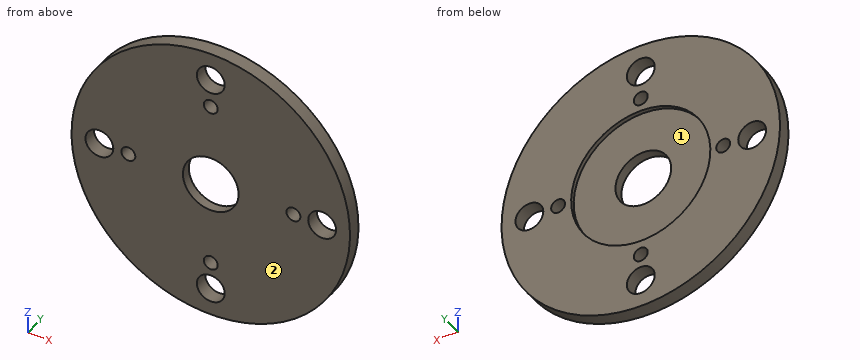
```python
from build123d import *

# Parameters (mm, degrees)
SKETCH1_R           = 10
SKETCH1_R_2         = 2
SKETCH1_R_3         = 1
SKETCH1_R_4         = 0.5
BOSS_EXTRUDE1_DEPTH = 1
SKETCH2_R           = 5
CUT_EXTRUDE1_DEPTH  = 0.3


with BuildPart() as part:
    # Sketch1 → Boss-Extrude1 (new body)
    with BuildSketch(Plane(origin=(0, 0, 0), x_dir=(1, 0, 0), z_dir=(0, 1, 0))):
        with Locations(Location((0, 0, 0), (0, 0, 270))):  # turned: the seam where the file's is
            Circle(SKETCH1_R)
        with Locations(Location((0, 0, 0), (0, 0, 270))):  # turned: the seam where the file's is
            Circle(SKETCH1_R_2, mode=Mode.SUBTRACT)
        with Locations(Location((-8, 0, 0), (0, 0, 270))):  # turned: the seam where the file's is
            Circle(SKETCH1_R_3, mode=Mode.SUBTRACT)
        with Locations(Location((-5.919172613, 0, 0), (0, 0, 270))):  # turned: the seam where the file's is
            Circle(SKETCH1_R_4, mode=Mode.SUBTRACT)
        with Locations(Location((0, -5.941415712, 0), (0, 0, 90))):  # turned: the seam where the file's is
            Circle(SKETCH1_R_4, mode=Mode.SUBTRACT)
        with Locations(Location((0, -8, 0), (0, 0, 90))):  # turned: the seam where the file's is
            Circle(SKETCH1_R_3, mode=Mode.SUBTRACT)
        with Locations(Location((5.936823246, 0, 0), (0, 0, 90))):  # turned: the seam where the file's is
            Circle(SKETCH1_R_4, mode=Mode.SUBTRACT)
        with Locations(Location((8, 0, 0), (0, 0, 90))):  # turned: the seam where the file's is
            Circle(SKETCH1_R_3, mode=Mode.SUBTRACT)
        with Locations(Location((0, 6.0333524, 0), (0, 0, 270))):  # turned: the seam where the file's is
            Circle(SKETCH1_R_4, mode=Mode.SUBTRACT)
        with Locations(Location((0, 8, 0), (0, 0, 270))):  # turned: the seam where the file's is
            Circle(SKETCH1_R_3, mode=Mode.SUBTRACT)
    extrude(amount=BOSS_EXTRUDE1_DEPTH)

    # Sketch2 → Cut-Extrude1 (cut)
    with BuildSketch(Plane(origin=(0, 1, 0), x_dir=(1, 0, 0), z_dir=(0, 1, 0))):
        with Locations(Location((0, 0, 0), (0, 0, 270))):  # turned: the seam where the file's is
            Circle(SKETCH2_R)
    extrude(amount=-CUT_EXTRUDE1_DEPTH, mode=Mode.SUBTRACT)


solid = part.part
```
Here's how the part is built. I have some questions about the finished solid (model axes, mm). Face numbers are marked on the shaded views. Coordinates: 2 decimals unless noted, no trailing zeros. Loops run counter-clockwise (first coordinate to the right, second up) from the corner with the lowest first, then second, coordinate; pieces in that order, holes last. Notation, with made-up numbers: M -30,58.5 L 17,58.5 A26 ccw 17,86.5 Z; hole C 63.25,7.5 d9. An arc over 180 degrees is marked long. One line per item, written item: value.
1. Imagine slicing it at A-A (x = -8). List the corners of the cut face in (y, z) for me, and give its area (3 significant figures).
Geometry says:
outline: M 0,-6 L 1,-6 L 1,-1 L 0,-1 Z; M 0,1 L 1,1 L 1,6 L 0,6 Z
area: 10.0 mm2
2. Will this pin go through, and if not, where does the flat tip stop? pin 1 Ø2.5 at (x, z) = (8, 0) entering from -Y.
Geometry says:
pin 1: stops at y = 0
3. Imagine slicing it at D-D (x = 0). List the corners of the cut face in (y, z) for me, and give its area (3 significant figures).
Geometry says:
outline: M 0,-10 L 1,-10 L 1,-9 L 0,-9 Z; M 0,-7 L 1,-7 L 1,-6.53 L 0,-6.53 Z; M 0,-5.53 L 1,-5.53 L 1,-5 L 0.7,-5 L 0.7,-2 L 0,-2 Z; M 0,2 L 0.7,2 L 0.7,5 L 1,5 L 1,5.44 L 0,5.44 Z; M 0,6.44 L 1,6.44 L 1,7 L 0,7 Z; M 0,9 L 1,9 L 1,10 L 0,10 Z
area: 8.20 mm2
4. Thinking about a two-plate mould opening in Z: for the marked faces 1 and 2, which applies, +Z half, -Z half, draft (parallel to the pull), parting line (faces both ways), or undercut?
Geometry says:
face 1: undercut
face 2: draft
5. Imagine slicing it at C-C (z = 8). List the corners of the cut face in (x, y) for me, and give its area (3 significant figures).
Geometry says:
outline: M -6,0 L -1,0 L -1,1 L -6,1 Z; M 1,0 L 6,0 L 6,1 L 1,1 Z
area: 10.0 mm2
6. Please list where these lines run through material, in increasing order: probe 1 along X at (y, z) = (0.3, 0); probe 2 along X at (y, z) = (0.8, 0); probe 3 along X at (y, z) = (0.95, -6).
Geometry says:
probe 1: x = -10 to -9, -7 to -6.42, -5.42 to -2, 2 to 5.44, 6.44 to 7, 9 to 10
probe 2: x = -10 to -9, -7 to -6.42, -5.42 to -5, 5 to 5.44, 6.44 to 7, 9 to 10
probe 3: x = -8 to -0.5, 0.5 to 8
7. Imagine slicing it at B-B (z = 0). List the corners of the cut face in (x, y) for me, and give its area (3 significant figures).
Geometry says:
outline: M -10,0 L -9,0 L -9,1 L -10,1 Z; M -7,0 L -6.42,0 L -6.42,1 L -7,1 Z; M -5.42,0 L -2,0 L -2,0.7 L -5,0.7 L -5,1 L -5.42,1 Z; M 2,0 L 5.44,0 L 5.44,1 L 5,1 L 5,0.7 L 2,0.7 Z; M 6.44,0 L 7,0 L 7,1 L 6.44,1 Z; M 9,0 L 10,0 L 10,1 L 9,1 Z
area: 8.20 mm2
